Design review of the part built by this model. Coordinates are the model's own, in mm. Give positions to 0.01 mm unless a question says otherwise; leave off trailing zeros. Loops run counter-clockwise (first coordinate to the right, second up) from the corner with the lowest first, then second, coordinate; pieces in that order, holes last. Notation, with made-up numbers: (75, 49) -> (125, 49) arc R25 ccw to (125, 76) -> close; hole circle Ø4 at (25.25, -29). An arc over 180 degrees is marked (long way). Answer as CSV lines item,"result".
from build123d import *

# Parameters (mm, degrees)
F0_R     = 7.778434
F0_R_2   = 7.877406
F1_DEPTH = 7


with BuildPart() as f1:
    # F0 (on Top) → F1 (new body)
    with BuildSketch(Plane.XY):
        with BuildLine():
            Line((-24.244773, 25.964786), (-34.002946, 39.3446))
            Line((-34.002946, 39.3446), (-34.002946, 0))
            Line((-34.002946, 0), (-24.244773, 13.379814))
            ThreePointArc((-24.244773, 13.379814), (-27.443761, 19.6723), (-24.244773, 25.964786))
        make_face()
        with BuildLine():
            Line((-5.30812, 0), (-5.30812, 39.3446))
            Line((-5.30812, 39.3446), (-15.066294, 25.964786))
            ThreePointArc((-15.066294, 25.964786), (-12.712963, 23.20178), (-11.867305, 19.6723))
            ThreePointArc((-11.867305, 19.6723), (-12.712963, 16.14282), (-15.066294, 13.379814))
            Line((-15.066294, 13.379814), (-5.30812, 0))
        make_face()
        with BuildLine():
            Line((-15.066294, 25.964786), (-5.30812, 39.3446))
            ThreePointArc((-5.30812, 39.3446), (-19.655533, 53.692013), (-34.002946, 39.3446))
            Line((-34.002946, 39.3446), (-24.244773, 25.964786))
            ThreePointArc((-24.244773, 25.964786), (-19.655533, 27.460528), (-15.066294, 25.964786))
        make_face()
        with Locations((-19.839631, 39.3446)):
            Circle(F0_R, mode=Mode.SUBTRACT)
        with BuildLine():
            ThreePointArc((-34.002946, 0), (-19.655533, -14.347413), (-5.30812, 0))
            Line((-5.30812, 0), (-15.066294, 13.379814))
            ThreePointArc((-15.066294, 13.379814), (-19.655533, 11.884072), (-24.244773, 13.379814))
            Line((-24.244773, 13.379814), (-34.002946, 0))
        make_face()
        with Locations((-19.655533, 0)):
            Circle(F0_R_2, mode=Mode.SUBTRACT)
    extrude(amount=F1_DEPTH)


solid = f1.part
Q1. We need section B-B, the plane x = -20. State the section outline as (y, z) points.
Filled sheet:
outline,"(-14.34, 0) -> (-7.87, 0) -> (-7.87, 7) -> (-14.34, 7) -> close; (7.87, 0) -> (11.89, 0) -> (11.89, 7) -> (7.87, 7) -> close; (27.45, 0) -> (31.57, 0) -> (31.57, 7) -> (27.45, 7) -> close; (47.12, 0) -> (53.69, 0) -> (53.69, 7) -> (47.12, 7) -> close"
Q2. We need section C-C, the plane y = -4. State the section outline as (x, z) points, and give its area (3 significant figures).
Filled sheet:
outline,"(-33.43, 0) -> (-26.44, 0) -> (-26.44, 7) -> (-33.43, 7) -> close; (-12.87, 0) -> (-5.88, 0) -> (-5.88, 7) -> (-12.87, 7) -> close"
area,"97.9 mm^2"
Q3. Clearance check with flat-ended pins moving along their axes: pin 1 Ø1 at (x, z) = (-14.5, 1) entering from +Y; pin 2 Ø1 at (y, z) = (-5.5, 5) entering from -X; pin 3 Ø4 at (x, z) = (-22, 5.5) entering from -Y. State where each tip first meets the part, or that it passes through.
Filled sheet:
pin 1,"stops at y = 52.92"
pin 2,"stops at x = -33.1"
pin 3,"stops at y = -14.34"
Q4. We need section D-D, the plane y = 6. State the section outline as (x, z) points, and give its area (3 significant figures).
Filled sheet:
outline,"(-34, 0) -> (-24.76, 0) -> (-24.76, 7) -> (-34, 7) -> close; (-14.55, 0) -> (-5.31, 0) -> (-5.31, 7) -> (-14.55, 7) -> close"
area,"129 mm^2"
Q5. The part is to be moulded in two halves that separate along X. For faces 1 (the flat face through (-26, 13, 0)), 2 (the cylindrical face through (-12.142, 2.366, 3.451)), 3 (the cylindrical face through (-26.01, 34.61, 3.45)), 4 (the cylindrical face through (-19.34, 53.69, 3.45)), say which applies: pulls with the +X half, pulls with the -X half, needs draft (parallel to the pull), parting line crosses it, or undercut.
Filled sheet:
face 1,"needs draft"
face 2,"undercut"
face 3,"undercut"
face 4,"parting line crosses it"
Q6. To check wall thickness, follow probe 1 along Y at (x, z) = (-19.75, 2); probe 2 along Y at (x, z) = (-26, 1.25); probe 3 along X at (y, z) = (3, 5.5). State the ranges of each line that lie inside material, in increasing order. Write a range as from..to.
Filled sheet:
probe 1,"y = -14.35..-7.88, 7.88..11.88, 27.46..31.57, 47.12..53.69"
probe 2,"y = -12.87..-4.67, 4.67..15.16, 24.19..34.6, 44.09..52.21"
probe 3,"x = -34..-26.94, -12.37..-5.31"
